Can you work these out from the model? Positions are in its coordinate system, mm. Coordinates: 2 decimals unless noted, no trailing zeros. Order: outer loops, then holes, each group sorted by start corner. A loop starts at its lowest first (then second) coordinate and runs counter-clockwise, first axis right, second up. Notation, with made-up numbers: (-28, 39) - (6, 39) arc R16 cw to (6, 66) - close; hole circle Ø6 at (-11.5, -30.5). An arc over 180 degrees is marked (long way). Use a Markdown table: item, result. Add a question column.
(1) I want a section at C-C (z = 5). List the corners of the cut face in (x, y) for me.
(2) If I drill on L1, parallel to Y at x = 0, z = 3; L2, parallel to Y at x = 0.75, z = 8; L3, parallel to X at y = 1.5, z = 6, over which ranges is the centre line in solid material (lowest first)? Write a range as [from, to].
(3) I want a section at B-B (x = 0). List the corners of the cut face in (y, z) for me, and give its area (3 significant figures).
(4) We'd pull the mould along Y, two halves only. Please class faces 1 (the flat face through (3, 0, 0)), 2 (the cylindrical face through (-3.972, 0.575, 4.095)), 3 (the cylindrical face through (5.723, 1.802, 3.372)): pulls with the +Y half, pulls with the -Y half, needs draft (parallel to the pull), parting line crosses it, or undercut.
(5) For pin 1 Ø4 at (y, z) = (-1, 2) entering from -X; pin 2 Ø3 at (x, y) = (0, 0) entering from -Z; pin 3 Ø5 at (x, z) = (4, 8.5) entering from -Y; pin 4 Ø1.5 at (y, z) = (-1, 8) entering from -X, each with a flat end and sliding along its axis, tell me the tip position at first contact or that it passes through.
(6) I want a section at A-A (y = 0). List the corners of the cut face in (x, z) for me, and give its area (3 significant figures).
(7) I want a section at D-D (z = 8.5). List the corners of the cut face in (x, y) for me.
```python
from build123d import *

# Parameters (mm, degrees)
SKICA1_R                 = 6
SKICA1_R_2               = 2.5
P_IDAT_VYSUNUT_M1_DEPTH  = 11
SKICA3_R                 = 1.5
ODEBRAT_VYSUNUT_M1_DEPTH = 11


with BuildPart() as part:
    # Skica1 → Přidat vysunutím1 (new body)
    with BuildSketch(Plane.XY):
        Circle(SKICA1_R)
        Circle(SKICA1_R_2, mode=Mode.SUBTRACT)
    extrude(amount=P_IDAT_VYSUNUT_M1_DEPTH)

    # Skica2 → Odebrat rotací1 (revolve, cut)
    with BuildSketch(Plane(origin=(0, 0, 0), x_dir=(0, 0, -1), z_dir=(1, 0, 0)), mode=Mode.PRIVATE) as odebrat_rotac_1_sk:
        with BuildLine():
            Line((-6.838910778, 6), (-9.5, 6))
            ThreePointArc((-9.5, 6), (-8.169455389, 5.25), (-6.838910778, 6))
        make_face()
    revolve(odebrat_rotac_1_sk.sketch.rotate(Axis((0, 0, 0), (0, 0, 1)), 90), axis=Axis((0, 0, 0), (0, 0, 1)), mode=Mode.SUBTRACT)

    # Skica3 → Odebrat vysunutím1 (cut)
    with BuildSketch(Plane(origin=(0, 0, 0), x_dir=(0, 0, -1), z_dir=(1, 0, 0))):
        with Locations(Location((-2.709871991, 0, 0), (0, 0, 180))):
            Circle(SKICA3_R)
    extrude(amount=-ODEBRAT_VYSUNUT_M1_DEPTH, mode=Mode.SUBTRACT)


solid = part.part
```
Answers follow:
| question | item | result |
|---|---|---|
| 1 | outline | circle Ø12 at (0, 0); hole circle Ø5 at (0, 0) |
| 2 | L1 | y = [-6, -2.5], [2.5, 6] |
| 2 | L2 | y = [-5.21, -2.38], [2.38, 5.21] |
| 2 | L3 | x = [-5.81, -2], [2, 5.81] |
| 3 | outline | (-6, 0) - (-2.5, 0) - (-2.5, 11) - (-6, 11) - (-6, 9.5) arc R1.56 cw to (-6, 6.84) - close; (2.5, 0) - (6, 0) - (6, 6.84) arc R1.56 cw to (6, 9.5) - (6, 11) - (2.5, 11) - close |
| 3 | area | 74.2 mm² |
| 4 | face 1 | needs draft |
| 4 | face 2 | undercut |
| 4 | face 3 | parting line crosses it |
| 5 | pin 1 | stops at x = -6 |
| 5 | pin 2 | passes through |
| 5 | pin 3 | stops at y = -5.75 |
| 5 | pin 4 | stops at x = -5.47 |
| 6 | outline | (-6, 0) - (-2.5, 0) - (-2.5, 1.21) - (-6, 1.21) - close; (-6, 4.21) - (-2.5, 4.21) - (-2.5, 11) - (-6, 11) - (-6, 9.5) arc R1.56 cw to (-6, 6.84) - close; (2.5, 0) - (6, 0) - (6, 6.84) arc R1.56 cw to (6, 9.5) - (6, 11) - (2.5, 11) - close |
| 6 | area | 63.7 mm² |
| 7 | outline | circle Ø10.57 at (0, 0); hole circle Ø5 at (0, 0) |
